Input: dimensioned drawing with shaded views. Units: mm. Origin: part minimum x, y, z. A direction names the side the tool comes from. Coordinates: 2 decimals unless noted, no trailing zeros. Order: outer loops, then holes, each group sorted by start corner. A loop starts at its lowest first (then second) coordinate and runs counter-clockwise, first axis right, second up. Notation, with made-up numbers: (80.5, 35) - (106.5, 35) arc R9 ccw to (106.5, 48) - close; hole circle Ø6 at (84.5, 1). An arc over 180 degrees is marked (long way). Answer as CSV lines item,"result". Start each with the question number.
Item 1: Section B-B (x = 25). Output: boundary loops of the cut face in (y, z), and give its area (3 significant figures).
Item 2: Draft query along X for the marked faces 1, 2 and 3. Return one class per face: +X half, -X half, draft (parallel to the pull), parting line (faces both ways), or undercut.
Item 3: Section D-D (y = 13). Output: boundary loops of the cut face in (x, z).
Item 4: Section C-C (z = 8). Output: boundary loops of the cut face in (x, y).
Item 5: First-contact query: pin 1 (8 mm diameter, centred on x = 27, y = 21, fed in from +Z); pin 2 (2 mm diameter, centred on x = 5, y = 31, fed in from +Z); pin 3 (3 mm diameter, centred on x = 25, y = 19, fed in from +Z); pin 4 (4 mm diameter, centred on x = 14, z = 14, fed in from +Y). Flat tips, straight axial feed; report the tip coordinate or a pass-through.
Item 6: Material intervals for line 1 along Y through (x, z) = (25, 11.75); line 2 along Y through (x, z) = (25, 14); line 3 along Z through (x, y) = (25, 10.4), sorted ascending.
Item 7: Section A-A (y = 19). Output: boundary loops of the cut face in (x, z).
Item 8: Access query for the marked faces 4 and 5. Directions: +Z, -Z, +X, -X, +Y, -Y. A direction counts if a zero-diameter tool reaches every point of the face in a straight line with its end or side. Return the directions, or none.
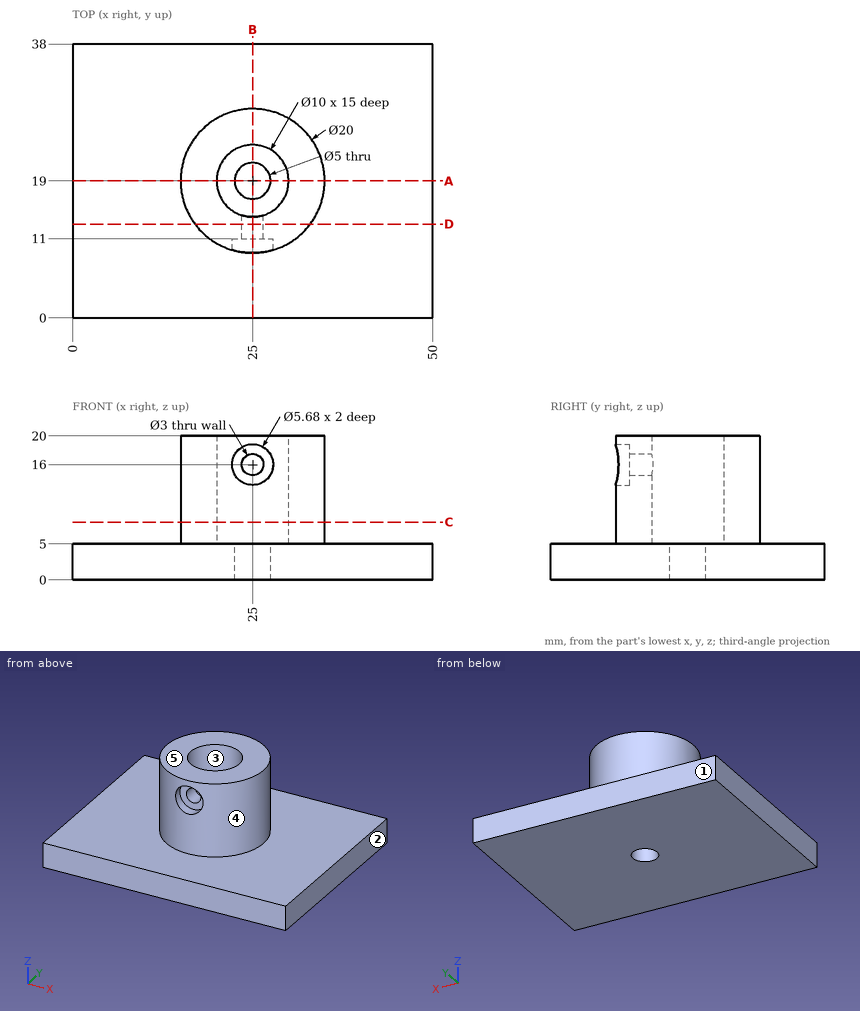
Determined:
1,outline,"(0, 0) - (16.5, 0) - (16.5, 5) - (14, 5) - (14, 14.5) - (11, 14.5) - (11, 13.16) - (9, 13.16) - (9, 5) - (0, 5) - close; (9, 18.84) - (11, 18.84) - (11, 17.5) - (14, 17.5) - (14, 20) - (9, 20) - close; (21.5, 0) - (38, 0) - (38, 5) - (29, 5) - (29, 20) - (24, 20) - (24, 5) - (21.5, 5) - close"
1,area,"295 mm^2"
2,face 1,"draft"
2,face 2,"+X half"
2,face 3,"undercut"
3,outline,"(0, 0) - (50, 0) - (50, 5) - (33, 5) - (33, 20) - (17, 20) - (17, 5) - (0, 5) - close; hole circle Ø3 at (25, 16)"
4,outline,"circle Ø20 at (25, 19); hole circle Ø10 at (25, 19)"
5,pin 1,"stops at z = 20"
5,pin 2,"stops at z = 5"
5,pin 3,"passes through"
5,pin 4,"stops at y = 23.36"
6,line 1,"y = 9 to 14, 24 to 29"
6,line 2,"y = 11 to 14, 24 to 29"
6,line 3,"z = 0 to 13.16, 18.84 to 20"
7,outline,"(0, 0) - (22.5, 0) - (22.5, 5) - (20, 5) - (20, 20) - (15, 20) - (15, 5) - (0, 5) - close; (27.5, 0) - (50, 0) - (50, 5) - (35, 5) - (35, 20) - (30, 20) - (30, 5) - (27.5, 5) - close"
8,face 4,"+Z"
8,face 5,"+Z, +X, -X, +Y, -Y"
